The listing builds one solid part. Answer for the finished solid, in the listing's coordinates (mm). A direction names the side the tool comes from. Give positions to 0.01 mm unless a question says otherwise; leave off trailing zeros. Order: outer loops, then holes, each group sorted by start corner. A loop starts at its lowest first (then second) coordinate and runs counter-clockwise, first axis right, second up.
```python
from build123d import *
from build123d import SkipClean  # not in build123d's __all__

# Parameters (mm, degrees)
F0_W     = 23
F0_H     = 12
F1_DEPTH = 22
F3_DEPTH = 4.5
F4_R     = 2.5
F5_DEPTH = 4
F6_R     = 2.5
F7_DEPTH = 2
F8_R     = 2.5
F9_DEPTH = 2.5


with BuildPart() as f1:
    # F0 (on Right) → F1 (new body)
    with BuildSketch(Plane.YZ):
        Rectangle(F0_W, F0_H)
    extrude(amount=F1_DEPTH)

    # F2 (on face) → F3 (join)
    with BuildSketch(Plane.YZ.offset(22)):
        with BuildLine():
            ThreePointArc((-5.5, -6), (-1.2573593129, -4.2426406871), (0.5, 0))
            ThreePointArc((0.5, 0), (-1.2573593129, 4.2426406871), (-5.5, 6))
            ThreePointArc((-5.5, 6), (-9.7426406871, 4.2426406871), (-11.5, 0))
            ThreePointArc((-11.5, 0), (-9.7426406871, -4.2426406871), (-5.5, -6))
        make_face()
    extrude(amount=F3_DEPTH)

    # F4 (on face) → F5 (join)
    with BuildSketch(Plane.YZ.offset(26.5)):
        with Locations((-5.5, 0)):
            Circle(F4_R)
    extrude(amount=F5_DEPTH)

    # F6 (on face) → F7 (join)
    with BuildSketch(Plane.YZ.offset(30.5)):
        with BuildLine():
            Line((-3.0505102572, -2.5), (9.5793642451, -1.9984247088))
            ThreePointArc((9.5793642451, -1.9984247088), (11.5, 0), (9.5793642451, 1.9984247088))
            Line((9.5793642451, 1.9984247088), (-3.0505102572, 2.5))
            ThreePointArc((-3.0505102572, 2.5), (-9, 0), (-3.0505102572, -2.5))
        make_face()
        with Locations((-5.5, 0)):
            Circle(F6_R, mode=Mode.SUBTRACT)
        with Locations((-5.5, 0)):
            Circle(F6_R)
    extrude(amount=F7_DEPTH)

    # F8 (on face) → F9 (join)
    with BuildSketch(Plane(origin=(30.5, 0, 0), x_dir=(0, -1, 0), z_dir=(-1, 0, 0))):
        with BuildLine():
            ThreePointArc((3.0505102572, -2.5), (6.8558735008, -3.2267021942), (9, 0))
            ThreePointArc((9, 0), (6.8558735008, 3.2267021942), (3.0505102572, 2.5))
            ThreePointArc((3.0505102572, 2.5), (2, 0), (3.0505102572, -2.5))
        make_face()
        with Locations((5.5, 0)):
            Circle(F8_R, mode=Mode.SUBTRACT)
    with SkipClean():  # cleaning this boolean's faces spoils the solid; the shape is the same uncleaned
        extrude(amount=F9_DEPTH)


solid = f1.part
```
1) Find section A-A (y = 8.25). Write down the section's boundary in (x, z).
Geometry says:
outline: (0, -6) - (22, -6) - (22, 6) - (0, 6) - close; (30.5, -2.05) - (32.5, -2.05) - (32.5, 2.05) - (30.5, 2.05) - close
2) Given P1, Ø1, axis at y = 6.5, z = 3.5, coming from the +X side; P2, Ø3, axis at y = -9.5, z = 3.5, coming from the +X side, each flat-ended and moving along its own axis, determine where each tip first touches the part or whether it passes through.
Geometry says:
P1: stops at x = 22
P2: stops at x = 26.5
3) For a pull along X with two mould halves and no side action, classify faces 4 (the flat face through (30.5, 4, 0)), 5 (the flat face through (11, 0, 6)), 6 (the flat face through (22, -10, -5)) as +X half, -X half, draft (parallel to the pull), parting line (faces both ways), or undercut.
Geometry says:
face 4: undercut
face 5: draft
face 6: +X half
4) Find section B-B (z = 1). Write down the section's boundary in (x, y).
Geometry says:
outline: (0, -11.5) - (22, -11.5) - (22, -11.42) - (26.5, -11.42) - (26.5, -7.79) - (28, -7.79) - (28, -8.85) - (32.5, -8.85) - (32.5, 11.23) - (30.5, 11.23) - (30.5, -2.15) - (28, -2.15) - (28, -3.21) - (26.5, -3.21) - (26.5, 0.42) - (22, 0.42) - (22, 11.5) - (0, 11.5) - close
5) Straight lines are drawn through the part: probe 1 along X at (y, z) = (0.25, -1.25); probe 2 along X at (y, z) = (7, -2); probe 3 along X at (y, z) = (-0.75, 3.5). For each, find the intervals that lie inside material, in ascending order.
Geometry says:
probe 1: x = 0 to 26.5, 30.5 to 32.5
probe 2: x = 0 to 22, 30.5 to 32.5
probe 3: x = 0 to 26.5
6) Find section C-C (y = -3.5). Write down the section's boundary in (x, z), then the cut area to 3 significant figures.
Geometry says:
outline: (0, -6) - (22, -6) - (22, -5.66) - (26.5, -5.66) - (26.5, -1.5) - (28, -1.5) - (28, -2.87) - (32.5, -2.87) - (32.5, 2.87) - (28, 2.87) - (28, 1.5) - (26.5, 1.5) - (26.5, 5.66) - (22, 5.66) - (22, 6) - (0, 6) - close
area: 345 mm2
7) A tool of negligible diameter and unlimited length cuts with its end or side. For faces 1 (the flat face through (22, -10, 5)), 2 (the cylindrical face through (31.5, 11.5, 0)), 3 (the flat face through (28, -3, 1)), from which of +Z, -Z, +X, -X, +Y, -Y can it reach the whole face along a straight path? Write none if from no direction.
Geometry says:
face 1: +Z, +X, -Y
face 2: +X, +Y
face 3: none
8) Find section D-D (x = 23). Write down the section's boundary in (y, z), then the cut area to 3 significant figures.
Geometry says:
outline: circle Ø12 at (-5.5, 0)
area: 113 mm2
